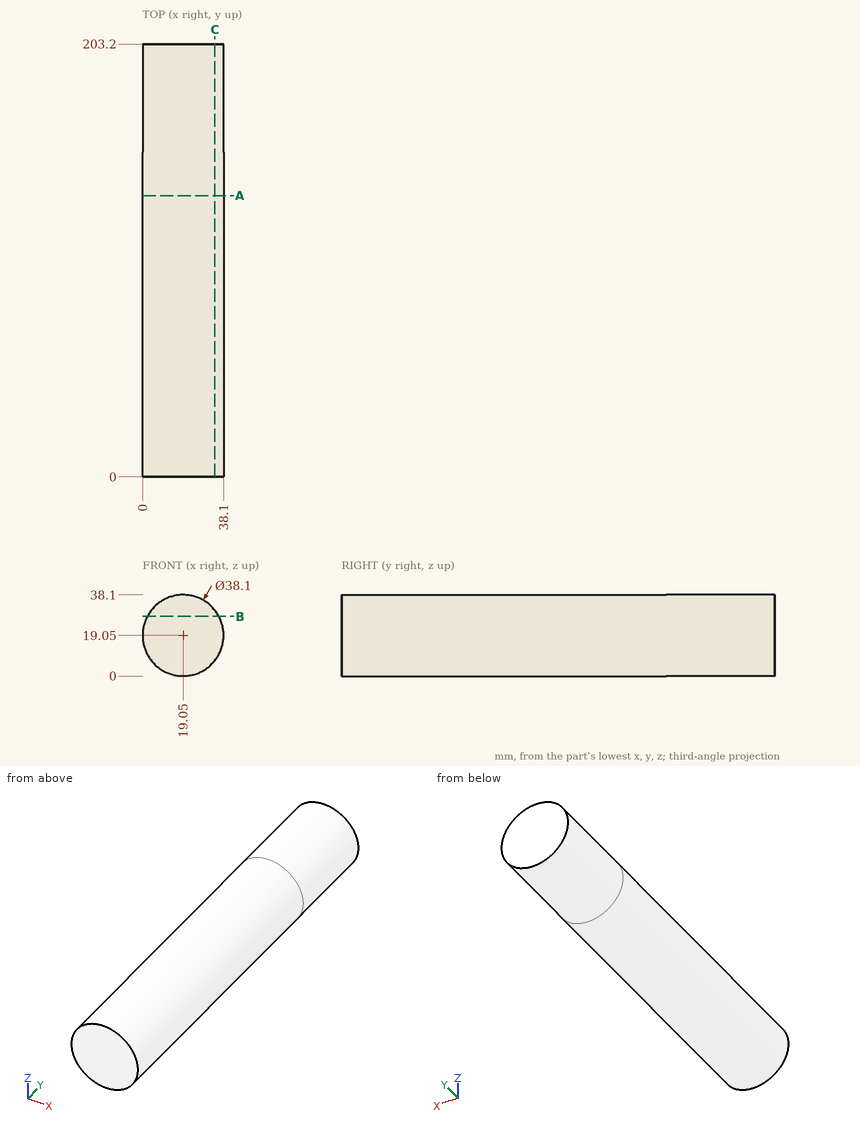
For this review, use the dimensioned drawing (mm, ordinates from the lowest corner) and the shaded views. Round coordinates to 2 decimals unless told otherwise and drop trailing zeros. Write each loop counter-clockwise with the first axis right and the second up, starting at its lowest first coordinate (ties: lowest second). Pieces come first, ordered by that corner, then holes. Notation, with made-up numbers: M 23,29 L 49,29 A31 cw 49,65 Z; hole C -23,-29.75 d2. An arc over 180 degrees is marked long. Write item = value, one per line. Start each with the question number.
(1) We need section C-C (x = 34). Give the boundary of the cut face in (y, z).
(2) We need section B-B (z = 28). Give the boundary of the cut face in (x, y), then the cut area to 3 significant figures.
(3) Clearance check with flat-ended pins moving along their axes: pin 1 Ø12 at (y, z) = (46.5, 31) entering from -X; pin 2 Ø2 at (x, z) = (12, 24) entering from -Y; pin 3 Ø5 at (x, y) = (20.5, 63) entering from +Z; pin 4 Ø1 at (y, z) = (31, 17) entering from +X. State where each tip first meets the part, or that it passes through.
(4) We need section A-A (y = 132). Give the boundary of the cut face in (x, z).
(5) For line 1 along X through (y, z) = (158, 20); line 2 along Z through (x, y) = (32, 151.5); line 3 along X through (y, z) = (168.5, 35), list the stretches that pass through material, from the lowest coordinate up.
Results found:
q1.outline = M 0,7.24 L 203.2,7.24 L 203.2,30.86 L 0,30.86 Z
q2.outline = M 2.23,0 L 35.87,0 L 35.87,203.2 L 2.23,203.2 Z
q2.area = 6,830 mm²
q3.pin_1 = 0.95
q3.pin_2 = 0
q3.pin_3 = 38.1
q3.pin_4 = 38.04
q4.outline = C 19.05,19.05 d38.1
q5.line_1 = 0.02 to 38.08
q5.line_2 = 5.08 to 33.02
q5.line_3 = 8.63 to 29.47
